```python
from build123d import *

# Parameters (mm, degrees)
EXTRUDE_1_DEPTH = 4
M2_5X0_45_1_D   = 2.05
FILLET_1_R      = 3


with BuildPart() as part:
    # 草图1 → 凸台-拉伸1 (new body)
    with BuildSketch(Plane.XY):
        with BuildLine():
            Line((0, -50), (-6, -50))
            Line((-6, -50), (-6, -46.111278447))
            ThreePointArc((-6, -46.111278447), (-12.001245585, -44.924604666), (-17.794779605, -42.960398262))
            ThreePointArc((-17.794779605, -42.960398262), (-20.187186997, -38.484518844), (-16.264045876, -35.264880132))
            Line((-16.264045876, -35.264880132), (16.264045876, -35.265962637))
            ThreePointArc((16.264045876, -35.265962637), (18.326373898, -35.838782605), (19.797870689, -37.393136741))
            Line((19.797870689, -37.393136741), (23.396904993, -44.188062152))
            ThreePointArc((23.396904993, -44.188062152), (12.053980513, -48.525267169), (0, -50))
        make_face()
    extrude(amount=EXTRUDE_1_DEPTH)

    # M2.5x0.45 螺纹孔1 (through all)
    with Locations(Plane(origin=(-4.11, -45.89, 4), x_dir=(1, 0, 0), z_dir=(0, 0, 1))):
        with Locations((0, 0)):
            Hole(M2_5X0_45_1_D / 2)

    # 圆角1
    fillet_1_edges = [part.edges().sort_by_distance(p)[0] for p in [
        (-6, -46.111278447, 2),
    ]]
    fillet(fillet_1_edges, radius=FILLET_1_R)


solid = part.part
```
The listing builds one solid part. Answer for the finished solid, in the listing's coordinates (mm). Give positions to 0.01 mm unless a question says otherwise; leave off trailing zeros. Loops run counter-clockwise (first coordinate to the right, second up) from the corner with the lowest first, then second, coordinate; pieces in that order, holes last. Notation, with made-up numbers: M -20,27.5 L -7,27.5 A26 ccw -7,64.5 Z; hole C 15.25,29.5 d2. An arc over 180 degrees is marked long. One line per item, written item: value.
Q1. Find the intervals of material crossed by line 1 (Y direction, x = -4.11, z = 2.15) (3 decimals); line 2 (X direction, y = -42.75, z = 2.75); line 3 (Y direction, x = -7, z = 2.45), in increasing order. Write a range as from..to.
Working result:
line 1: y = -50..-46.915, -44.865..-35.265
line 2: x = -18.23..22.64
line 3: y = -46.44..-35.27
Q2. A cutting plane is placed at B-B on x = -4.11. Determine the outline of the cut face in (y, z) (3 decimals), then the cut area to 3 significant figures.
Working result:
outline: M -50,0 L -46.915,0 L -46.915,4 L -50,4 Z; M -44.865,0 L -35.265,0 L -35.265,4 L -44.865,4 Z
area: 50.7 mm^2
Q3. A cutting plane is placed at C-C on y = -38.25. Determine the outline of the cut face in (x, z).
Working result:
outline: M -20.13,0 L 20.25,0 L 20.25,4 L -20.13,4 Z
Q4. Determine the mould class of faces 1 (the face through (-3.977, -44.874, 1.972)), 2 (the face through (-6, -49, 2)), 3 (the face through (21.57, -40.74, 1.97)) for opening direction X: +X half, -X half, draft (parallel to the pull), parting line (faces both ways), or undercut.
Working result:
face 1: undercut
face 2: -X half
face 3: +X half
Q5. A cutting plane is placed at A-A on z = 3.1. Determine the outline of the cut face in (x, y) (3 decimals), then the cut area to 3 significant figures.
Working result:
outline: M -17.795,-42.96 A46.5 ccw -8.455,-45.725 A3 cw -6,-48.675 L -6,-50 L 0,-50 A50 ccw 23.397,-44.188 L 19.798,-37.393 A3.999 ccw 16.264,-35.266 L -16.264,-35.265 A4 ccw Z; hole C -4.11,-45.89 d2.05
area: 491 mm^2
Q6. A cutting plane is placed at D-D on x = 10.5. Determine the outline of the cut face in (y, z).
Working result:
outline: M -48.89,0 L -35.27,0 L -35.27,4 L -48.89,4 Z
Q7. Flat-ended cylindrical pins translate along their axes: P1, Ø1, axis at y = -40, z = 2.5, coming from the -X side; P2, Ø1.1, axis at y = -49, z = 2, coming from the -X side. Find the tip coordinate at first contact, or state that the pin passes through.
Working result:
P1: stops at x = -20.26
P2: stops at x = -6.01
